Work out the finished part from the listing and answer in its coordinate system (mm). Coordinates: 2 decimals unless noted, no trailing zeros. Use CSV: the item, a comma, the result in double quotes. Start each with the question number.
Autodesk Inventor part; units mm, degrees
ref_plane "YZ Plane" through (0, 0, 0) normal (1, 0, 0) x (0, 1, 0)
ref_plane "XZ Plane" through (0, 0, 0) normal (0, 1, 0) x (-1, 0, 0)
ref_plane "XY Plane" through (0, 0, 0) normal (0, 0, 1) x (1, 0, 0)
sketch "스케치1" plane through (0, 0, 0) normal (0, 0, 1) x (1, 0, 0)
  line L0 (-19.5, -10) -> (19.5, -10)
  line L1 (20, -9.5) -> (20, 9.5)
  line L2 (19.5, 10) -> (-19.5, 10)
  line L3 (-20, 9.5) -> (-20, -9.5)
  circle A0 centre (-17, 7) radius 2
  line L4 (0, -12.143) -> (0, 11.1651)
  line L5 (28.9925, 0) -> (-24.8769, 0)
  circle A1 centre (-10, 0) radius 2.1
  line L6 (-10, 12.7543) -> (-10, -12.5913)
  line L7 (10, -12.5913) -> (10, 12.7543)
  circle A2 centre (10, 0) radius 2.1
  line L8 (-12.65, -10) -> (-12.65, -8.5)
  line L9 (-12.65, -8.5) -> (-14.15, -8.5)
  line L10 (-14.15, -8.5) -> (-14.15, -4.7403)
  line L11 (-5.85, -4.7397) -> (-5.85, -8.5)
  line L12 (-5.85, -8.5) -> (-7.35, -8.5)
  line L13 (-7.35, -8.5) -> (-7.35, -10)
  arc A3 (-5.85, -4.7397) -> (-14.15, -4.7403) centre (-9.9996, -10) ccw
  line L14 (-10, -3.05) -> (-10.25, -3.3047)
  line L15 (-10, -3.05) -> (-9.7398, -3.305)
  line L16 (12.65, -10) -> (12.65, -8.5)
  line L17 (12.65, -8.5) -> (14.15, -8.5)
  line L18 (14.15, -8.5) -> (14.15, -4.7403)
  line L19 (5.85, -4.7397) -> (5.85, -8.5)
  line L20 (5.85, -8.5) -> (7.35, -8.5)
  line L21 (7.35, -8.5) -> (7.35, -10)
  arc A4 (14.15, -4.7403) -> (5.85, -4.7397) centre (9.9996, -10) ccw
  line L22 (10, -3.05) -> (10.25, -3.3047)
  line L23 (10, -3.05) -> (9.7398, -3.305)
  line L24 (-20, 2.65) -> (-18.5, 2.65)
  line L25 (-18.5, 2.65) -> (-18.5, 4.15)
  line L26 (-18.5, 4.15) -> (-14.7403, 4.15)
  line L27 (-14.7397, -4.15) -> (-18.5, -4.15)
  line L28 (-18.5, -4.15) -> (-18.5, -2.65)
  line L29 (-18.5, -2.65) -> (-20, -2.65)
  line L30 (-13.05, 0) -> (-13.305, -0.2602)
  line L31 (-13.05, 0) -> (-13.3047, 0.25)
  arc A5 (-14.7397, -4.15) -> (-14.7403, 4.15) centre (-20, -0.0004) ccw
  line L32 (-7.35, 10) -> (-7.35, 8.5)
  line L33 (-7.35, 8.5) -> (-5.85, 8.5)
  line L34 (-5.85, 8.5) -> (-5.85, 4.7403)
  line L35 (-14.15, 4.7397) -> (-14.15, 8.5)
  line L36 (-14.15, 8.5) -> (-12.65, 8.5)
  line L37 (-12.65, 8.5) -> (-12.65, 10)
  line L38 (-10, 3.05) -> (-10.2602, 3.305)
  line L39 (-10, 3.05) -> (-9.75, 3.3047)
  arc A6 (-14.15, 4.7397) -> (-5.85, 4.7403) centre (-10.0004, 10) ccw
  line L40 (14.7397, -4.15) -> (18.5, -4.15)
  line L41 (18.5, -4.15) -> (18.5, -2.65)
  line L42 (18.5, -2.65) -> (20, -2.65)
  arc A7 (14.7403, 4.15) -> (14.7397, -4.15) centre (20, -0.0004) ccw
  line L43 (20, 2.65) -> (18.5, 2.65)
  line L44 (18.5, 2.65) -> (18.5, 4.15)
  line L45 (18.5, 4.15) -> (14.7403, 4.15)
  line L46 (13.05, 0) -> (13.305, -0.2602)
  line L47 (13.05, 0) -> (13.3047, 0.25)
  line L48 (14.15, 4.7397) -> (14.15, 8.5)
  line L49 (14.15, 8.5) -> (12.65, 8.5)
  line L50 (12.65, 8.5) -> (12.65, 10)
  arc A8 (5.85, 4.7403) -> (14.15, 4.7397) centre (10.0004, 10) ccw
  line L51 (7.35, 10) -> (7.35, 8.5)
  line L52 (7.35, 8.5) -> (5.85, 8.5)
  line L53 (5.85, 8.5) -> (5.85, 4.7403)
  line L54 (10, 3.05) -> (10.2602, 3.305)
  line L55 (10, 3.05) -> (9.75, 3.3047)
  circle A9 centre (-17, -7) radius 2
  circle A10 centre (17, 7) radius 2
  circle A11 centre (17, -7) radius 2
  line L56 (-3.85, -8.5) -> (3.85, -8.5)
  line L57 (3.85, 8.5) -> (-3.85, 8.5)
  line L58 (-4.35, -8.5) -> (4.35, 8.5) construction
  line L59 (4.35, -8.5) -> (-4.35, 8.5) construction
  arc A12 (-3.85, 8.5) -> (-4.35, 8) centre (-3.85, 8) ccw
  arc A13 (4.35, 8) -> (3.85, 8.5) centre (3.85, 8) ccw
  arc A14 (3.85, -8.5) -> (4.35, -8) centre (3.85, -8) ccw
  arc A15 (-4.35, -8) -> (-3.85, -8.5) centre (-3.85, -8) ccw
  line L60 (-4.35, 8) -> (-4.35, 4.1325)
  line L61 (-4.35, -4.3275) -> (-4.35, -8)
  line L62 (4.35, -8) -> (4.35, -4.3275)
  line L63 (4.35, 4.3275) -> (4.35, 8)
  arc A16 (4.4769, -3.9946) -> (4.4769, 3.9946) centre (0, 0) ccw
  arc A17 (-4.35, 4.1325) -> (-4.4769, -3.9946) centre (0, 0) ccw
  arc A18 (-4.35, -4.3275) -> (-4.4769, -3.9946) centre (-4.85, -4.3275) ccw
  arc A19 (4.35, 4.3275) -> (4.4769, 3.9946) centre (4.85, 4.3275) ccw
  arc A20 (4.4769, -3.9946) -> (4.35, -4.3275) centre (4.85, -4.3275) ccw
  arc A21 (-19.5, 10) -> (-20, 9.5) centre (-19.5, 9.5) ccw
  arc A22 (-20, -9.5) -> (-19.5, -10) centre (-19.5, -9.5) ccw
  arc A23 (19.5, -10) -> (20, -9.5) centre (19.5, -9.5) ccw
  arc A24 (20, 9.5) -> (19.5, 10) centre (19.5, 9.5) ccw
  point P0 (20, 10)
  point P1 (20, -10)
  point P2 (-20, 10)
  point P3 (-14.15, -6.6202)
  point P4 (-12.65, -9.25)
  point P5 (-10.0001, -3.3)
  point P6 (14.15, -6.6202)
  point P7 (12.65, -9.25)
  point P8 (10.0001, -3.3)
  point P9 (-19.25, 2.65)
  point P10 (-16.6202, 4.15)
  point P11 (-13.3, 0.0001)
  point P12 (-7.35, 9.25)
  point P13 (-5.85, 6.6202)
  point P14 (-9.9999, 3.3)
  point P15 (13.3, 0.0001)
  point P16 (19.25, 2.65)
  point P17 (16.6202, 4.15)
  point P18 (22.5913, 0)
  point P19 (9.9999, 3.3)
  point P20 (7.35, 9.25)
  point P21 (5.85, 6.6202)
  point P22 (10, 12.5913)
  point P23 (-5.85, -6.6199)
  point P24 (-4.35, -4.1325)
  point P25 (4.35, -4.1325)
  point P26 (4.35, 4.1325)
  point P27 (4.35, 6.1638)
  point P28 (-4.35, 6.0662)
  dimension "d0" = 40
  dimension "d1" = 20
  dimension "d2" = 4
  dimension "d3" = 34
  dimension "d4" = 14
  dimension "d5" = 4.2
  dimension "d6" = 20
  dimension "d8" = 4.2
  dimension "d9" = 20
  dimension "d12" = 1.5
  dimension "d13" = 6.7
  dimension "d14" = 8.3
  dimension "d15" = 5.3
  dimension "d16" = 5.3
  dimension "d17" = 8.3
  dimension "d18" = 6.7
  dimension "d19" = 0.5
  dimension "d20" = 0.25
  dimension "d23" = 180
  dimension "d27" = 180
  dimension "d29" = 1.5
  dimension "d31" = 1.5
  dimension "d32" = 0.5
  dimension "d33" = 0.5
  dimension "d34" = 0.5
  dimension "d35" = 8.7
extrude "돌출1" add sketch "스케치1" along normal blind 600 contours A22 L3 L29 L28 L27 A5 L30 L5 A1 L6 L14 A3 L10 L9 L8 L0 | L13 L12 L11 A3 L15 L6 A1 L5 A17 A18 L61 A15 L56 L4 L0 | L4 L56 A14 L62 A20 A16 L5 A2 L7 L23 A4 L19 L20 L21 L0 | L3 A21 L2 L37 L36 L35 A6 L38 L6 A1 L5 L31 A5 L26 L25 L24 | A1 L6 L39 A6 L34 L33 L32 L2 L4 L57 A12 L60 A17 L5 | L16 L17 L18 A4 L22 L7 A2 L5 L46 A7 L40 L41 L42 L1 A23 L0 | L4 L2 L51 L52 L53 A8 L55 L7 A2 L5 A16 A19 L63 A13 L57 | L7 L54 A8 L48 L49 L50 L2 A24 L1 L43 L44 L45 A7 L47 L5 A2
equation "\"d8\" = d5"
properties part number "20x40 profile"
1) The part is cut by section A-A on z = 502. State how many separate pieces and enclosed holes the cut face has, plus the area to 3 significant figures.
2) Straight lines are drawn through the part: line 1 (Y direction, x = 17.5, z = 530.5); line 2 (X direction, y = -0.25, z = 348) (3 decimals); line 3 (Y direction, x = 17, z = 396). For each, find the intervals that lie inside material, in ascending order. Write a range as [from, to].
3) A flat-ended cylindrical pin translates along its axis: P1, Ø1, axis at y = -2, z = 480.5, coming from the -X side. Find the tip coordinate at first contact, or state that the pin passes through.
Answer key:
1,separate pieces,"1"
1,enclosed holes,"7"
1,area,"271 mm^2"
2,line 1,"[-10, -8.94], [-5.06, -4.15], [4.15, 5.06], [8.94, 10]"
2,line 2,"[-13.295, -12.085], [-7.915, -5.995], [5.995, 7.915], [12.085, 13.295]"
2,line 3,"[-10, -9], [-5, -4.15], [4.15, 5], [9, 10]"
3,P1,"x = -13.78"
